from build123d import *

# Parameters (mm, degrees)
SKETCH_1_W                   = 22.4
SKETCH_1_H                   = 12.5
EXTRUDE_1_DEPTH              = 3.5
HOLE_WIZARD_M2_2_D           = 2.4
HOLE_WIZARD_M2_2_CBORE_D     = 4.4
HOLE_WIZARD_M2_2_CBORE_DEPTH = 2


with BuildPart() as part:
    # 草图1 → 凸台-拉伸1 (new body)
    with BuildSketch(Plane(origin=(0, 0, 0), x_dir=(1, 0, 0), z_dir=(0, 1, 0))):
        Polygon((-36, -9.25), (0, -9.25), (23, -9.25), (23, 9.25), (0, 9.25), (-36, 9.25), align=None)
        with Locations((-18, 0)):
            Rectangle(SKETCH_1_W, SKETCH_1_H, mode=Mode.SUBTRACT)
    extrude(amount=EXTRUDE_1_DEPTH)

    # M2 凹头盖螺钉的柱形沉头孔2 (through all)
    with Locations(Plane(origin=(-31.85, 3.5, 0), x_dir=(0, 0, 1), z_dir=(0, 1, 0))):
        with Locations((0, 0), (0, 27.7)):
            CounterBoreHole(HOLE_WIZARD_M2_2_D / 2, HOLE_WIZARD_M2_2_CBORE_D / 2, HOLE_WIZARD_M2_2_CBORE_DEPTH)


solid = part.part
The model under review builds one solid part; all positions refer to its coordinate system, in mm. A direction names the side the tool comes from. Coordinates: 2 decimals unless noted, no trailing zeros. Write each loop counter-clockwise with the first axis right and the second up, starting at its lowest first coordinate (ties: lowest second). Pieces come first, ordered by that corner, then holes. Notation, with made-up numbers: (72, -14) - (125, -14) arc R12 cw to (125, -8) - close; hole circle Ø8 at (57.25, -26). An arc over 180 degrees is marked (long way). Answer as a JSON object with one key per item and string values. Group by question number.
1. Add section A-A (x = -12.5). Give the boundary of the cut face in (y, z), plus the area to 3 significant figures.
2. To check wall thickness, follow probe 1 along X at (y, z) = (2, 0); probe 2 along X at (y, z) = (1.05, 0); probe 3 along X at (y, z) = (2.3, 6). State the ranges of each line that lie inside material, in increasing order.
3. Add section B-B (z = -3.75). Give the boundary of the cut face in (x, y).
4. Machinability: for faces 1 (the face through (-29.2, 2, 0)), 2 (the face through (-2.295, 2.514, 1.183)), 3 (the face through (23, 2, 0)), which of the approach directions +Z, -Z, +X, -X, +Y, -Y give a long, thin tool a straight path to every point of the face, cutting with its end or side? Answer none if there is none.
5. Add section C-C (z = 0). Give the boundary of the cut face in (x, y), plus the area to 3 significant figures.
6. Mouldability with a two-part tool opening along X and no side actions: class faces 4 (the face through (-7, 2, 9.25)), 5 (the face through (-6, 1.5, 0)), 6 (the face through (-36, 2, 0)) as pulls with the +X half, pulls with the -X half, needs draft (parallel to the pull), parting line crosses it, or undercut.
7. Clearance check with flat-ended pins moving along their axes: pin 1 Ø8 at (x, z) = (14, -5) entering from -Y; pin 2 Ø2 at (x, z) = (-31.85, 0) entering from +Y; pin 3 Ø1.3 at (x, z) = (-32, 1) entering from +Y. State where each tip first meets the part, or that it passes through.
8. Add section D-D (x = -31.85). Give the boundary of the cut face in (y, z).
Findings:
{
 "1": {"outline": "(0, -9.25) - (3.5, -9.25) - (3.5, -6.25) - (0, -6.25) - close; (0, 6.25) - (3.5, 6.25) - (3.5, 9.25) - (0, 9.25) - close", "area": "21.0 mm²"},
 "2": {"probe 1": "-36 to -34.05, -29.65 to -29.2, -6.8 to -6.35, -1.95 to 23", "probe 2": "-36 to -33.05, -30.65 to -29.2, -6.8 to -5.35, -2.95 to 23", "probe 3": "-36 to -29.2, -6.8 to 23"},
 "3": {"outline": "(-36, 0) - (-29.2, 0) - (-29.2, 3.5) - (-36, 3.5) - close; (-6.8, 0) - (23, 0) - (23, 3.5) - (-6.8, 3.5) - close"},
 "4": {"face 1": "+Y, -Y", "face 2": "+Y", "face 3": "+Z, -Z, +X, +Y, -Y"},
 "5": {"outline": "(-36, 0) - (-33.05, 0) - (-33.05, 1.5) - (-34.05, 1.5) - (-34.05, 3.5) - (-36, 3.5) - close; (-30.65, 0) - (-29.2, 0) - (-29.2, 3.5) - (-29.65, 3.5) - (-29.65, 1.5) - (-30.65, 1.5) - close; (-6.8, 0) - (-5.35, 0) - (-5.35, 1.5) - (-6.35, 1.5) - (-6.35, 3.5) - (-6.8, 3.5) - close; (-2.95, 0) - (23, 0) - (23, 3.5) - (-1.95, 3.5) - (-1.95, 1.5) - (-2.95, 1.5) - close", "area": "103 mm²"},
 "6": {"face 4": "needs draft", "face 5": "undercut", "face 6": "pulls with the -X half"},
 "7": {"pin 1": "y = 0", "pin 2": "through", "pin 3": "y = 1.5"},
 "8": {"outline": "(0, -9.25) - (3.5, -9.25) - (3.5, -2.2) - (1.5, -2.2) - (1.5, -1.2) - (0, -1.2) - close; (0, 1.2) - (1.5, 1.2) - (1.5, 2.2) - (3.5, 2.2) - (3.5, 9.25) - (0, 9.25) - close"}
}
